Input: dimensioned drawing with shaded views. Units: mm. Origin: part minimum x, y, z. A direction names the side the tool comes from. Coordinates: 2 decimals unless noted, no trailing zeros. Loops run counter-clockwise (first coordinate to the right, second up) from the corner with the lowest first, then second, coordinate; pieces in that order, holes last. Notation, with made-up numbers: (46.25, 40.5) -> (92.25, 40.5) arc R15 ccw to (92.25, 49.5) -> close; hole circle Ø7 at (86, -24.5). An arc over 180 degrees is marked (long way). Answer as CSV lines item,"result".
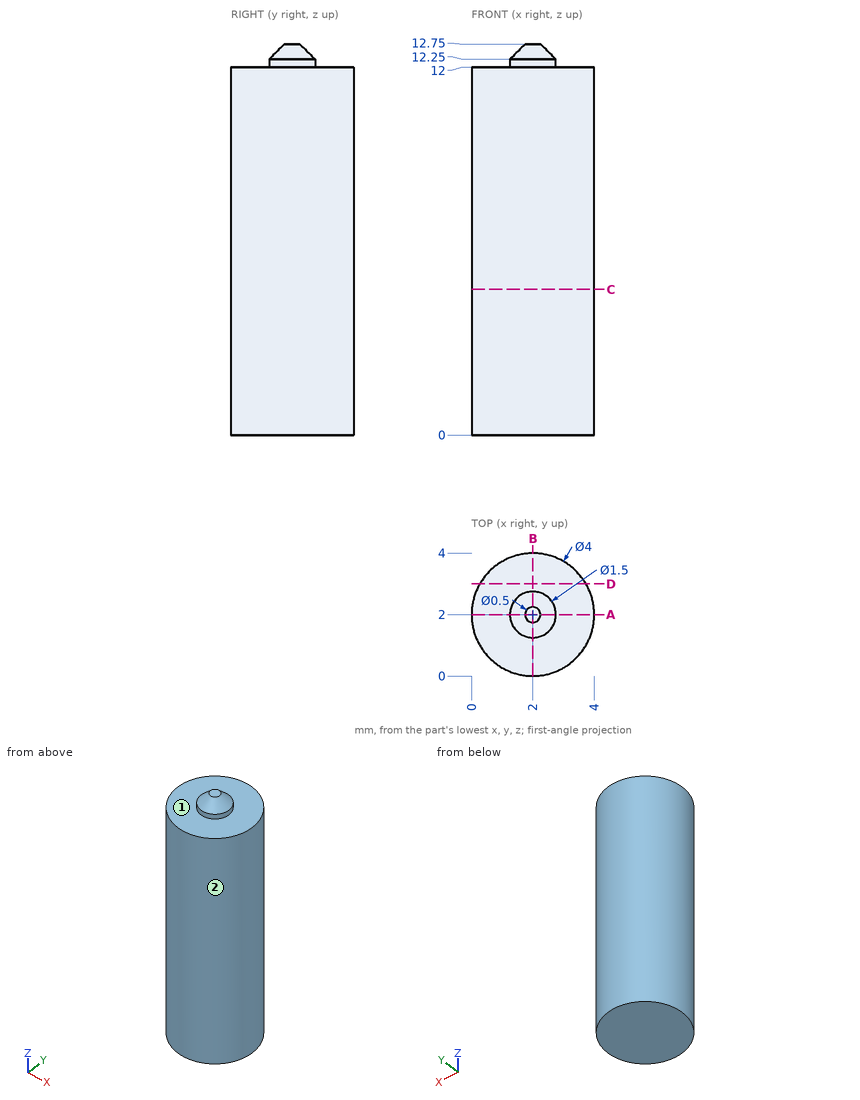
(1) Material intervals for L1, parallel to X at y = 2.1, z = 1.25; L2, parallel to Z at x = 3, y = 1.5, sorted ascending. Write a range as [from, to].
Computed values:
L1,"[0, 4]"
L2,"[0, 12]"
(2) Cut plane A-A (y = 2). Return the cut outline in (x, z).
Computed values:
outline,"(0, 0) -> (4, 0) -> (4, 12) -> (2.75, 12) -> (2.75, 12.25) -> (2.25, 12.75) -> (1.75, 12.75) -> (1.25, 12.25) -> (1.25, 12) -> (0, 12) -> close"
(3) Access query for the marked faces 1 and 2. Directions: +Z, -Z, +X, -X, +Y, -Y. A direction counts if a zero-diameter tool reaches every point of the face in a straight line with its end or side. Return the directions, or none.
Computed values:
face 1,"+Z"
face 2,"+Z, -Z"
(4) Cut plane C-C (z = 4.75). Return the cut outline in (x, y).
Computed values:
outline,"circle Ø4 at (2, 2)"
(5) Cut plane D-D (y = 3). Return the cut outline in (x, z).
Computed values:
outline,"(0.27, 0) -> (3.73, 0) -> (3.73, 12) -> (0.27, 12) -> close"
(6) Pin query (flat end, axial travel): pin 1 Ø1.5 at (y, z) = (1, 3.5) entering from +X. Return the tip coordinate at first contact, or that it passes through.
Computed values:
pin 1,"x = 3.98"
